Input: dimensioned drawing with shaded views. Units: mm. Origin: part minimum x, y, z. Round coordinates to 2 decimals unless told otherwise and drop trailing zeros. Order: outer loops, then holes, each group sorted by start corner. A loop starts at its lowest first (then second) coordinate and runs counter-clockwise, first axis right, second up. Notation, with made-up numbers: M -22,36 L 34,36 A13 ccw 34,54 Z; hole C 48.5,-12.75 d1. An arc over 180 degrees is marked long. Use CSV: the item, a comma, the result in double quotes. Start each with the question number.
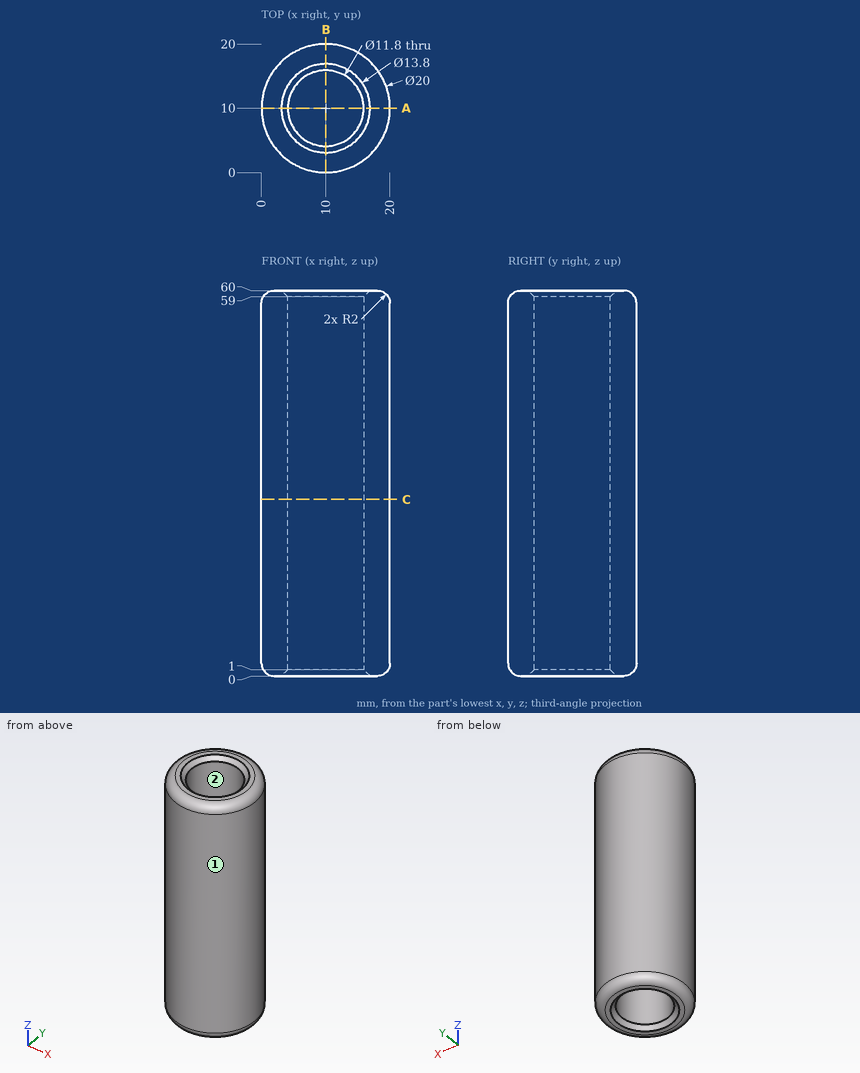
(1) Contact query for flat-ended pins moving along their axis: P1, Ø1, axis at x = 8.5, z = 13, coming from the +Y side; P2, Ø8, axis at x = 5, z = 42.5, coming from the -Y side; P3, Ø1.5, axis at y = 4.5, z = 19, coming from the +X side. Output: stop coordinate, or through.
(2) Draft query along Y for the marked faces 1 and 2. Return one class per face: pulls with the +Y half, pulls with the -Y half, needs draft (parallel to the pull), parting line crosses it, or undercut.
(3) Section C-C on z = 27.5. Return loops of the section in (x, y).
(4) Line query: line 1 along Y through (x, z) = (10, 46.5); line 2 along Z through (x, y) = (5.25, 1.5); line 3 along X through (y, z) = (10.5, 31). Output: solid intervals per line, ascending.
(5) Section A-A on y = 10. Return loops of the section in (x, z).
Results below:
1,P1,"stops at y = 19.95"
1,P2,"stops at y = 0.05"
1,P3,"stops at x = 18.8"
2,face 1,"parting line crosses it"
2,face 2,"undercut"
3,outline,"C 10,10 d20; hole C 10,10 d11.8"
4,line 1,"y = 0 to 4.1, 15.9 to 20"
4,line 2,"z = 1.01 to 58.99"
4,line 3,"x = 0.01 to 4.12, 15.88 to 19.99"
5,outline,"M 0,2 A2 ccw 2,0 L 3.1,0 L 4.1,1 L 4.1,59 L 3.1,60 L 2,60 A2 ccw 0,58 Z; M 15.9,1 L 16.9,0 L 18,0 A2 ccw 20,2 L 20,58 A2 ccw 18,60 L 16.9,60 L 15.9,59 Z"
